from build123d import *

# Parameters (mm, degrees)
CHAMFER1_SIZE = 0.3


with BuildPart() as part:
    # Sketch1 → Revolve1 (revolve)
    with BuildSketch(Plane(origin=(0, 0, 0), x_dir=(0, 0, -1), z_dir=(1, 0, 0))):
        Polygon((-2.94, 11.945), (2.94, 11.945), (5.115, 9.77), (5.115, 7.987), (0.5, 7.987), (0.5, 6.945), (-0.5, 6.945), (-0.5, 7.987), (-5.115, 7.987), (-5.115, 9.77), align=None)
    revolve(axis=Axis((0, 0, 5.115), (0, 0, -1)))

    # Chamfer1
    chamfer1_edges = [part.edges().sort_by_distance(p)[0] for p in [
        (0, -7.987, 5.115),
        (0, -7.987, -5.115),
    ]]
    chamfer(chamfer1_edges, length=CHAMFER1_SIZE)


solid = part.part
Input: part model. Units: mm. Frame: model coordinates. A direction names the side the tool comes from. Round coordinates to 2 decimals unless told otherwise and drop trailing zeros. Loops run counter-clockwise (first coordinate to the right, second up) from the corner with the lowest first, then second, coordinate; pieces in that order, holes last. Notation, with made-up numbers: (-28.5, 44) -> (29.5, 44) arc R35 cw to (29.5, 83) -> close; hole circle Ø10 at (56.5, -38). An arc over 180 degrees is marked (long way). Answer as a JSON object with one key per item and string values. Group by question number.
1) Reachability of faces 1 (the cylindrical face through (5.398, -5.887, 2.688)), 2 (the cylindrical face through (-7.27, -9.48, -0.04)), 3 (the cylindrical face through (5.398, -5.887, -2.627)) from +Z, -Z, +X, -X, +Y, -Y: full face, straight path, thin tool, end or side. Return the list, or none.
2) Section query D-D on z = -1.75. Output: boundary loops of the cut face in (x, y) (3 decimals).
3) Ray query, L1, parallel to X at y = 0, z = -0.25 (3 decimals); L2, parallel to X at y = 0, z = -2.9 (3 decimals); L3, parallel to Y at x = 3.25, z = -4. Return the intervals inside material, ascending.
4) Section query A-A on x = 0. Output: boundary loops of the cut face in (y, z) (3 decimals).
5) Section query C-C on z = 0. Output: boundary loops of the cut face in (x, y) (3 decimals), plus the area to 3 significant figures.
6) Pin query (flat end, axial travel): pin 1 (4 mm diameter, centred on x = -7, z = 1, fed in from +Y); pin 2 (2 mm diameter, centred on x = -3.5, z = 3, fed in from +Y); pin 3 (3 mm diameter, centred on x = -2.5, z = 2.5, fed in from +Y). Return the tip coordinate at first contact, or that it passes through.
7) Draft query along Y for faces 4 (the conical face through (2.976, 9.449, 4.979)), 5 (the flat face through (-7.2, 4.4, 5.115)), 6 (the cylindrical face through (-6.78, -1.51, 0.01)). Return one class per face: +Y half, -Y half, draft (parallel to the pull), parting line (faces both ways), or undercut.
Reply:
{
 "1": {"face 1": "+Z", "face 2": "+Z, -Z", "face 3": "-Z"},
 "2": {"outline": "circle Ø23.89 at (0, 0); hole circle Ø15.974 at (0, 0)"},
 "3": {"L1": "x = -11.945 to -6.945, 6.945 to 11.945", "L2": "x = -11.945 to -7.987, 7.987 to 11.945", "L3": "y = -10.39 to -7.3, 7.3 to 10.39"},
 "4": {"outline": "(-11.945, -2.94) -> (-9.77, -5.115) -> (-8.287, -5.115) -> (-7.987, -4.815) -> (-7.987, -0.5) -> (-6.945, -0.5) -> (-6.945, 0.5) -> (-7.987, 0.5) -> (-7.987, 4.815) -> (-8.287, 5.115) -> (-9.77, 5.115) -> (-11.945, 2.94) -> close; (6.945, -0.5) -> (7.987, -0.5) -> (7.987, -4.815) -> (8.287, -5.115) -> (9.77, -5.115) -> (11.945, -2.94) -> (11.945, 2.94) -> (9.77, 5.115) -> (8.287, 5.115) -> (7.987, 4.815) -> (7.987, 0.5) -> (6.945, 0.5) -> close"},
 "5": {"outline": "circle Ø23.89 at (0, 0); hole circle Ø13.89 at (0, 0)", "area": "297 mm2"},
 "6": {"pin 1": "stops at y = 10.85", "pin 2": "stops at y = 11.68", "pin 3": "stops at y = 11.9"},
 "7": {"face 4": "parting line", "face 5": "draft", "face 6": "undercut"}
}
